Build history of the part. All positions in model axes, mm. Face numbers are marked on the shaded views. Give positions to 0.01 mm unless a question says otherwise; leave off trailing zeros. Loops run counter-clockwise (first coordinate to the right, second up) from the corner with the lowest first, then second, coordinate; pieces in that order, holes last. Notation, with made-up numbers: M 12,4.5 L 34,4.5 A32 ccw 34,38.5 Z; hole C 39.25,71.5 d6. An arc over 180 degrees is marked long. Answer as a JSON object with one key per item and string values. Group by question number.
1. Drop a flat-ended pin along its axis: pin 1 Ø10 at (x, z) = (-28.5, 58) entering from -Y. Give the stop position or say it passes through.
2. Slice it at C-C (x = -10). List the corners of the cut face in (y, z), then the cut area to 3 significant figures.
3. Slice it at B-B (z = 103). List the corners of the cut face in (x, y).
4. Slice it at A-A (y = -14.5). List the corners of the cut face in (x, z).
5. Mould opens along X. For the marked faces 1, 2, 3 and 4 say: released by +X, released by -X, zero draft, split by the parting line, or undercut.
6. Drill centre lines: line 1 along Z through (x, y) = (-45.5, 43.5); line 2 along X through (y, z) = (15.5, 27); line 3 along Y through (x, z) = (38.5, 106). Where is each one in solid material? Low to high. Write a range as [from, to].
from build123d import *

# Parameters (mm, degrees)
F0_W      = 101.6
F0_H      = 101.6
F1_DEPTH  = 127
F2_T      = -2.54
F4_R      = 1.5875
F5_DEPTH  = 7.62
F11_DEPTH = 10.16


with BuildPart() as f1:
    # F0 (on Top) → F1 (new body)
    with BuildSketch(Plane.XY):
        Rectangle(F0_W, F0_H)
    extrude(amount=F1_DEPTH)

    # F2
    f2_openings = [f1.faces().sort_by_distance(p)[0] for p in [
        (0, -50.8, 63.5),
    ]]
    offset(amount=F2_T, openings=f2_openings)

    # F4 (on face) → F5 (join)
    with BuildSketch(Plane(origin=(48.26, 0, 0), x_dir=(0, -1, 0), z_dir=(-1, 0, 0))):
        with Locations((37.686419, 9.374908)):
            Circle(F4_R)
    extrude(amount=F5_DEPTH)

    # F7: F1 across plane


with BuildPart() as f1_1:
    add(f1.part)
    add(f1.part.mirror(Plane.YZ))

    # F8: F1 across plane


with BuildPart() as f1_2:
    add(f1_1.part)
    add(f1_1.part.mirror(Plane.YZ))

    # F10 (on face) → F11 (join)
    with BuildSketch(Plane(origin=(-50.8, 0, 0), x_dir=(0, -1, 0), z_dir=(-1, 0, 0))):
        with BuildLine():
            ThreePointArc((25.4, 17.4625), (26.522532, 17.927468), (26.9875, 19.05))
            ThreePointArc((26.9875, 19.05), (24.277468, 20.172532), (25.4, 17.4625))
        make_face()
    extrude(amount=-F11_DEPTH)

    # F12: F1 across plane


with BuildPart() as f1_3:
    add(f1_2.part)
    add(f1_2.part.mirror(Plane.YZ))


solid = f1_3.part
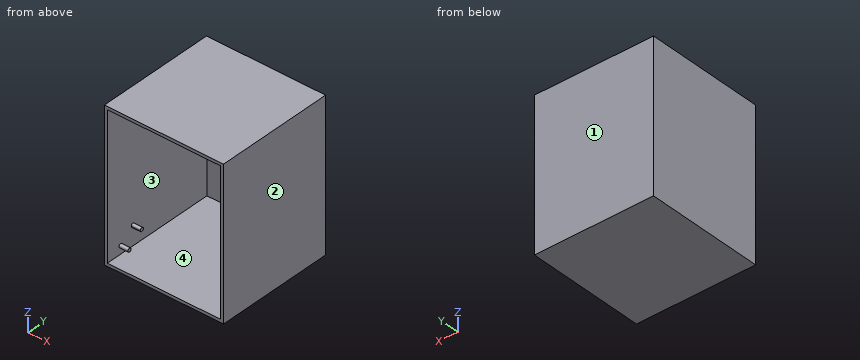
Established:
{
 "1": {"pin 1": "stops at y = 48.26"},
 "2": {"outline": "M -50.8,0 L 50.8,0 L 50.8,127 L -50.8,127 L -50.8,124.46 L 48.26,124.46 L 48.26,2.54 L -50.8,2.54 Z", "area": "826 mm^2"},
 "3": {"outline": "M -50.8,-50.8 L -48.26,-50.8 L -48.26,48.26 L 48.26,48.26 L 48.26,-50.8 L 50.8,-50.8 L 50.8,50.8 L -50.8,50.8 Z"},
 "4": {"outline": "M -50.8,0 L 50.8,0 L 50.8,127 L -50.8,127 Z; hole M -48.26,2.54 L 48.26,2.54 L 48.26,124.46 L -48.26,124.46 Z"},
 "5": {"face 1": "zero draft", "face 2": "released by +X", "face 3": "undercut", "face 4": "undercut"},
 "6": {"line 1": "z = [0, 2.54], [124.46, 127]", "line 2": "x = [-50.8, -48.26], [48.26, 50.8]", "line 3": "y = [48.26, 50.8]"}
}
